```python
from build123d import *

# Parameters (mm, degrees)
CUT_EXTRUDE1_DEPTH = 0.75
FILLET1_R          = 0.125


with BuildPart() as part:
    # Sketch1 → Revolve1 (revolve)
    with BuildSketch(Plane(origin=(0, 0, 0), x_dir=(0, 0, -1), z_dir=(1, 0, 0))):
        with BuildLine():
            Line((0, 1.5), (-1.5, 1.5))
            ThreePointArc((-1.5, 1.5), (-1.978515811, 0.925250119), (-2.3, 0.25))
            Line((-2.3, 0.25), (-2.155662433, 0))
            Line((-2.155662433, 0), (-1, 0))
            Line((-1, 0), (-1, -16))
            Line((-1, -16), (0, -16))
            Line((0, -16), (0, 1.5))
        make_face()
    revolve(axis=Axis((0, -16, 0), (0, 1, 0)))

    # Sketch2 → Cut-Extrude1 (cut)
    with BuildSketch(Plane(origin=(0, 1.5, 0), x_dir=(1, 0, 0), z_dir=(0, 1, 0))):
        Polygon((0, 1.154700538), (-1, 0.577350269), (-1, -0.577350269), (0, -1.154700538), (1, -0.577350269), (1, 0.577350269), align=None)
    extrude(amount=-CUT_EXTRUDE1_DEPTH, mode=Mode.SUBTRACT)

    # Fillet1
    fillet1_edges = [part.edges().sort_by_distance(p)[0] for p in [
        (0.5, 1.5, -0.866025404),
        (-0.5, 1.5, -0.866025404),
        (-1, 1.5, 0),
        (-0.5, 1.5, 0.866025404),
        (0.5, 1.5, 0.866025404),
        (1, 1.5, 0),
        (0, 1.5, -1.5),
    ]]
    fillet(fillet1_edges, radius=FILLET1_R)


solid = part.part
```
Source: CAD feature listing. Evaluate the final solid. Frame: model axes, mm. Give positions to 0.01 mm unless a question says otherwise; leave off trailing zeros. Loops run counter-clockwise (first coordinate to the right, second up) from the corner with the lowest first, then second, coordinate; pieces in that order, holes last. Notation, with made-up numbers: (75, -8.75) -> (123, -8.75) arc R5 cw to (123, -0.75) -> close; hole circle Ø1 at (37.5, -14.75). An arc over 180 degrees is marked (long way). Use a Markdown table: item, result. Add a question column.
(1) Section query A-A (y = -0.25). Output: boundary loops of the cut face in (x, z).
(2) First-contact query: pin 1 Ø1.5 at (y, z) = (-7, -1) entering from +X; pin 2 Ø1.5 at (x, y) = (-1.5, -10.5) entering from +Z; pin 3 Ø0.5 at (y, z) = (1, 0) entering from +X. Flat tips, straight axial feed; report the tip coordinate or a pass-through.
(3) Ray query, line 1 (Y direction, x = -0.45, z = -1.05); line 2 (Y direction, x = -0.3, z = -0.4); line 3 (X direction, y = -9.75, z = 0.7). Return the intervals inside material, ascending.
(4) Pull-direction query (Z, two-part tool) for faces 1 (the face through (1, 0, 1)), 2 (the face through (-1, -8, 0)), 3 (the face through (0, 0.75, 0)); classes: +Z half, -Z half, draft (parallel to the pull), parting line (faces both ways), or undercut.
Checked values:
| question | item | result |
|---|---|---|
| 1 | outline | circle Ø2 at (0, 0) |
| 2 | pin 1 | x = 0.97 |
| 2 | pin 2 | z = 0.66 |
| 2 | pin 3 | x = 2.08 |
| 3 | line 1 | 0 to 1.5 |
| 3 | line 2 | -16 to 0.75 |
| 3 | line 3 | -0.71 to 0.71 |
| 4 | face 1 | draft |
| 4 | face 2 | parting line |
| 4 | face 3 | undercut |
